Input: part model. Units: mm. Frame: model coordinates. Give positions to 0.01 mm unless a question says otherwise; leave off trailing zeros. Loops run counter-clockwise (first coordinate to the right, second up) from the corner with the lowest first, then second, coordinate; pieces in that order, holes last. Notation, with made-up numbers: M -2.75,57 L 44.25,57 A27 cw 44.25,94 Z; hole C 12.25,36.5 d7. An arc over 180 degrees is marked long. Use CSV: the item, a comma, the result in double quotes. Start each with the question number.
Q1. Material intervals for line 1 along X through (y, z) = (6.75, 0); line 2 along X through (y, z) = (6.25, -3); line 3 along Z through (x, y) = (-3.5, 1.5), sorted ascending.
Q2. Section A-A, the plane x = 0. Output: boundary loops of the cut face in (y, z).
Q3. Pin query (flat end, axial travel): pin 1 (1.5 mm diameter, centred on x = -6.5, y = 1.5, fed in from +Z); pin 2 (2 mm diameter, centred on x = -7, y = 1, fed in from -Z); pin 3 (1.5 mm diameter, centred on y = 3.5, z = -4, fed in from -X); pin 4 (5 mm diameter, centred on x = 0, z = 0, fed in from -Y). Return the tip coordinate at first contact, or that it passes through.
Q4. Section B-B, the plane z = 0. Output: boundary loops of the cut face in (x, y).
Q5. Pull-direction query (X, two-part tool) for faces 1 (the cylindrical face through (-10.74, 3.95, -2.38)), 2 (the flat face through (0, 0, 5)), 3 (the cylindrical face through (-3.905, 4.198, -0.867)); classes: released by +X, released by -X, zero draft, split by the parting line, or undercut.
Q6. Section C-C, the plane y = 2. Output: boundary loops of the cut face in (x, z), plus the area to 3 significant figures.
from build123d import *

# Parameters (mm, degrees)
SKETCH1_R           = 11
SKETCH1_R_2         = 4
BOSS_EXTRUDE1_DEPTH = 8
CHAMFER1_SIZE       = 0.5


with BuildPart() as part:
    # Sketch1 → Boss-Extrude1 (new body)
    with BuildSketch(Plane(origin=(0, 0, 0), x_dir=(1, 0, 0), z_dir=(0, 1, 0))):
        with Locations(Location((0, 0, 0), (0, 0, 270))):
            Circle(SKETCH1_R)
        with Locations(Location((0, 0, 0), (0, 0, 270))):
            Circle(SKETCH1_R_2, mode=Mode.SUBTRACT)
    extrude(amount=BOSS_EXTRUDE1_DEPTH)

    # Chamfer1
    chamfer1_edges = [part.edges().sort_by_distance(p)[0] for p in [
        (0, 0, -11),
        (0, 8, -11),
        (0, 0, -4),
    ]]
    chamfer(chamfer1_edges, length=CHAMFER1_SIZE)


solid = part.part
A:
1,line 1,"-11 to -4, 4 to 11"
1,line 2,"-10.58 to -2.65, 2.65 to 10.58"
1,line 3,"-10.43 to -1.94, 1.94 to 10.43"
2,outline,"M 0,-10.5 L 0.5,-11 L 7.5,-11 L 8,-10.5 L 8,-4 L 0.5,-4 L 0,-4.5 Z; M 0,4.5 L 0.5,4 L 8,4 L 8,10.5 L 7.5,11 L 0.5,11 L 0,10.5 Z"
3,pin 1,"z = 9.38"
3,pin 2,"z = -9.22"
3,pin 3,"x = -10.51"
3,pin 4,"through"
4,outline,"M -11,0.5 L -10.5,0 L -4.5,0 L -4,0.5 L -4,8 L -10.5,8 L -11,7.5 Z; M 4,0.5 L 4.5,0 L 10.5,0 L 11,0.5 L 11,7.5 L 10.5,8 L 4,8 Z"
5,face 1,"split by the parting line"
5,face 2,"zero draft"
5,face 3,"undercut"
6,outline,"C 0,0 d22; hole C 0,0 d8"
6,area,"330 mm^2"
